Autodesk Inventor part; units mm, degrees
ref_plane "YZ Plane" through (0, 0, 0) normal (1, 0, 0) x (0, 1, 0)
ref_plane "XZ Plane" through (0, 0, 0) normal (0, 1, 0) x (-1, 0, 0)
ref_plane "XY Plane" through (0, 0, 0) normal (0, 0, 1) x (1, 0, 0)
sketch "Sketch1" plane through (0, 0, 0) normal (1, 0, 0) x (0, 1, 0)
  line L0 (0, 0) -> (-4, 0)
  line L1 (0, 0) -> (36, 0)
  line L2 (36, 0) -> (36, -50)
  line L3 (36, -50) -> (0, -50)
  line L4 (0, -50) -> (0, 0)
  line L5 (-4, 0) -> (-4, -10)
  line L6 (-4, -20) -> (-4, -30)
  line L7 (0, -20) -> (0, -10)
  line L8 (-4, -10) -> (0, -10)
  line L9 (0, -20) -> (-4, -20)
  line L10 (-4, -40) -> (-4, -50)
  line L11 (0, -40) -> (0, -30)
  line L12 (-4, -30) -> (0, -30)
  line L13 (0, -40) -> (-4, -40)
  line L14 (-4, -50) -> (0, -50)
  dimension "d230" = 36
  dimension "d231" = 50
  dimension "d236" = 10
  dimension "d240" = 10
  dimension "d241" = 4
extrude "Extrusion1" add sketch "Sketch1" against normal blind 4
properties part number "Langbektang houder"
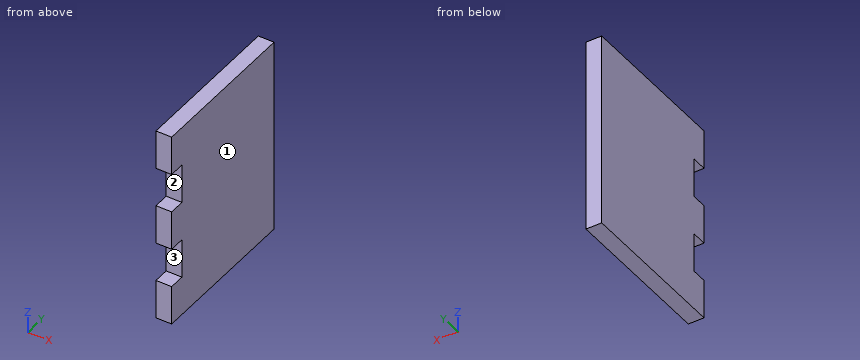
Can you work these out from the model? Positions are in its coordinate system, mm. Face numbers are marked on the shaded views. Coordinates: 2 decimals unless noted, no trailing zeros. Order: outer loops, then holes, each group sorted by start corner. A loop starts at its lowest first (then second) coordinate and runs counter-clockwise, first axis right, second up. Notation, with made-up numbers: (-11.75, 4) - (37.25, 4) arc R11 cw to (37.25, 18) - close; hole circle Ø7 at (42, 0). An arc over 180 degrees is marked (long way). Answer in a Markdown table with one row per item.
1. For pin 1 (1.2 mm diameter, centred on x = -1.5, z = -15.5, fed in from -Y); pin 2 (1 mm diameter, centred on y = 3, z = -24, fed in from +X), each with a flat end and sliding along its axis, tell me the tip position at first contact or that it passes through.
Reply:
| item | result |
|---|---|
| pin 1 | stops at y = 0 |
| pin 2 | stops at x = 0 |
2. If we mould it in two halves opening along Z, with no side actions, what happens to the marked faces 1, 2 and 3? For each: pulls with the +Z half, pulls with the -Z half, needs draft (parallel to the pull), parting line crosses it, or undercut.
Reply:
| item | result |
|---|---|
| face 1 | needs draft |
| face 2 | undercut |
| face 3 | undercut |
3. If I drill on line 1 along Y through (x, z) = (-2.7, -34.5), over which ranges is the centre line in solid material (lowest first)?
Reply:
| item | result |
|---|---|
| line 1 | y = 0 to 36 |
4. Suppose I cut it at A-A (x = -1.7). Please give me the cut outline in (y, z), and give its area (3 significant figures).
Reply:
| item | result |
|---|---|
| outline | (-4, -50) - (36, -50) - (36, 0) - (-4, 0) - (-4, -10) - (0, -10) - (0, -20) - (-4, -20) - (-4, -30) - (0, -30) - (0, -40) - (-4, -40) - close |
| area | 1,920 mm^2 |
5. Suppose I cut it at B-B (z = -18.5). Please give me the cut outline in (x, y), and give its area (3 significant figures).
Reply:
| item | result |
|---|---|
| outline | (-4, 0) - (0, 0) - (0, 36) - (-4, 36) - close |
| area | 144 mm^2 |
